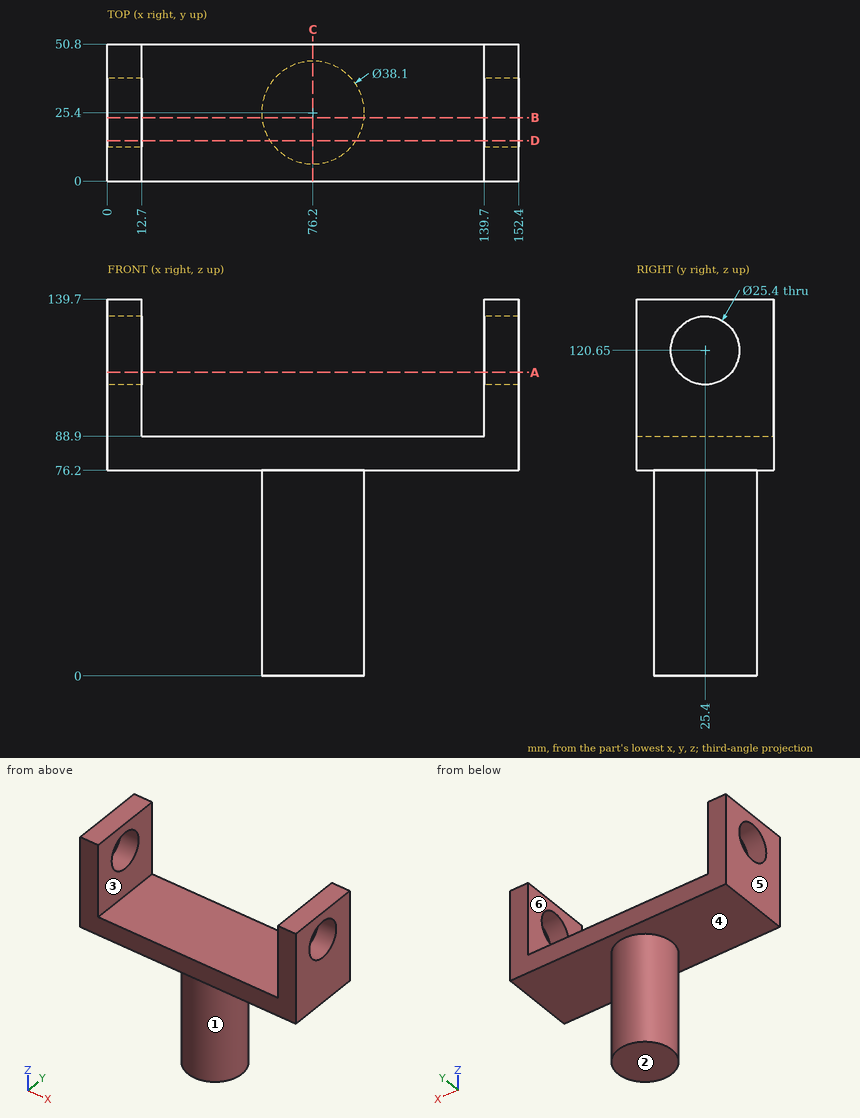
Geometry: see drawing. Coordinates: mm, zero at the bounding-box minimum. A direction names the side the tool comes from. Coordinates: 2 decimals unless noted, no trailing zeros. Loops run counter-clockwise (first coordinate to the right, second up) from the corner with the lowest first, then second, coordinate; pieces in that order, holes last.
(1) Section B-B on y = 23.5. Return the cut outline in (x, z).
(2) Section A-A on z = 112.5. Return the cut outline in (x, y).
(3) First-contact query: pin 1 Ø10 at (x, z) = (88.5, 25) entering from +Y; pin 2 Ø2 at (x, y) = (112, 11) entering from +Z; pin 3 Ø12 at (y, z) = (29, 66) entering from -X; pin 4 Ø15 at (y, z) = (31, 109.5) entering from -X. Flat tips, straight axial feed; report the tip coordinate or a pass-through.
(4) Set-up query: the marked faces 1, 2 and 3. Return all of +Z, -Z, +X, -X, +Y, -Y with unobstructed straight access to the full face (end or side cutting, diameter ignored); none if empty.
(5) Section D-D on y = 15. Return the cut outline in (x, z), then the cut area to 3 significant figures.
(6) Section C-C on x = 76.2. Return the cut outline in (y, z).
(7) Material intervals for probe 1 along X at (y, z) = (29.5, 103); probe 2 along Z at (x, y) = (5, 25.4); probe 3 along Z at (x, y) = (49.5, 33), sorted ascending.
(8) Pull-direction query (X, two-part tool) for the marked faces 4, 5 and 6; classes: released by +X, released by -X, zero draft, split by the parting line, or undercut.
Data:
1. outline: (0, 76.2) - (57.24, 76.2) - (57.24, 0) - (95.16, 0) - (95.16, 76.2) - (152.4, 76.2) - (152.4, 108.09) - (139.7, 108.09) - (139.7, 88.9) - (12.7, 88.9) - (12.7, 108.09) - (0, 108.09) - close; (0, 133.21) - (12.7, 133.21) - (12.7, 139.7) - (0, 139.7) - close; (139.7, 133.21) - (152.4, 133.21) - (152.4, 139.7) - (139.7, 139.7) - close
2. outline: (0, 0) - (12.7, 0) - (12.7, 15.66) - (0, 15.66) - close; (0, 35.14) - (12.7, 35.14) - (12.7, 50.8) - (0, 50.8) - close; (139.7, 0) - (152.4, 0) - (152.4, 15.66) - (139.7, 15.66) - close; (139.7, 35.14) - (152.4, 35.14) - (152.4, 50.8) - (139.7, 50.8) - close
3. pin 1: stops at y = 43
3. pin 2: stops at z = 88.9
3. pin 3: stops at x = 57.15
3. pin 4: stops at x = 0
4. face 1: -Z
4. face 2: -Z, +X, -X, +Y, -Y
4. face 3: +Z, +Y, -Y
5. outline: (0, 76.2) - (60.24, 76.2) - (60.24, 0) - (92.16, 0) - (92.16, 76.2) - (152.4, 76.2) - (152.4, 113.36) - (139.7, 113.36) - (139.7, 88.9) - (12.7, 88.9) - (12.7, 113.36) - (0, 113.36) - close; (0, 127.94) - (12.7, 127.94) - (12.7, 139.7) - (0, 139.7) - close; (139.7, 127.94) - (152.4, 127.94) - (152.4, 139.7) - (139.7, 139.7) - close
5. area: 5,290 mm2
6. outline: (0, 76.2) - (6.35, 76.2) - (6.35, 0) - (44.45, 0) - (44.45, 76.2) - (50.8, 76.2) - (50.8, 88.9) - (0, 88.9) - close
7. probe 1: x = 0 to 12.7, 139.7 to 152.4
7. probe 2: z = 76.2 to 107.95, 133.35 to 139.7
7. probe 3: z = 76.2 to 88.9
8. face 4: zero draft
8. face 5: released by -X
8. face 6: undercut
